Job drawing, mm, ordinate dimensions from the low corner. One solid piece. A direction names the side the tool comes from. Give positions to 0.01 mm unless a question says otherwise; leave off trailing zeros. Loops run counter-clockwise (first coordinate to the right, second up) from the corner with the lowest first, then second, coordinate; pieces in that order, holes last. Notation, with made-up numbers: M 77,42.25 L 88,42.25 A30 ccw 88,68.25 Z; hole C -30,1.25 d9. An arc over 180 degrees is marked long. One line per question, with ' | ' between items.
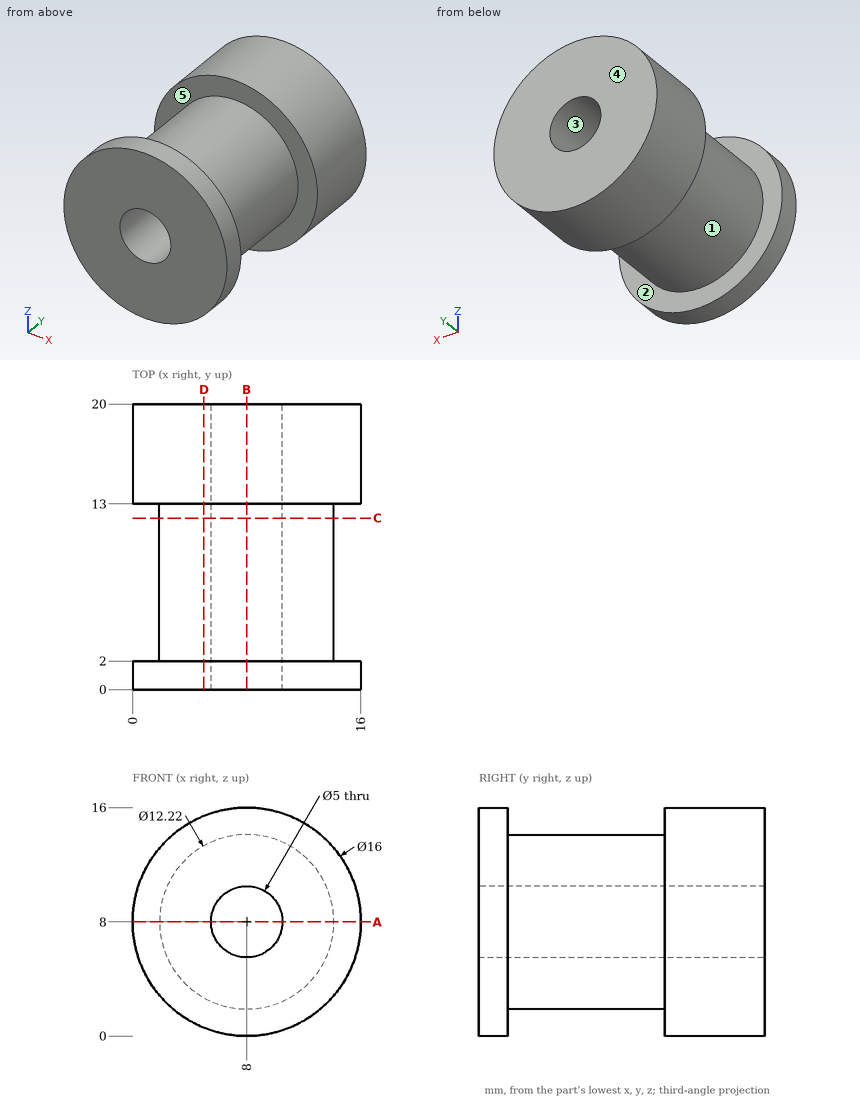
Item 1: Saw through at C-C on y = 12. Give the cut face in (x, z).
Conclusion:
outline: C 8,8 d12.22; hole C 8,8 d5
Item 2: Saw through at A-A on z = 8. Give the cut face in (x, y).
Conclusion:
outline: M 0,0 L 5.5,0 L 5.5,20 L 0,20 L 0,13 L 1.89,13 L 1.89,2 L 0,2 Z; M 10.5,0 L 16,0 L 16,2 L 14.11,2 L 14.11,13 L 16,13 L 16,20 L 10.5,20 Z
Item 3: Saw through at D-D on x = 5. Give the cut face in (y, z).
Conclusion:
outline: M 0,0.58 L 2,0.58 L 2,2.68 L 13,2.68 L 13,0.58 L 20,0.58 L 20,15.42 L 13,15.42 L 13,13.32 L 2,13.32 L 2,15.42 L 0,15.42 Z
Item 4: 3-axis set-ups, long thin cutter, end or side, ignore diameter. For the marked faces 4 and 5: which of +Z, -Z, +X, -X, +Y, -Y reach the whole face in a straight line?
Conclusion:
face 4: +Z, -Z, +X, -X, +Y | face 5: none
Item 5: Mould opens along X. For the marked faces 1, 2 and 3 say: pulls with the +X half, pulls with the -X half, needs draft (parallel to the pull), parting line crosses it, or undercut.
Conclusion:
face 1: parting line crosses it | face 2: needs draft | face 3: undercut
Item 6: Saw through at B-B on x = 8. Give the cut face in (y, z).
Conclusion:
outline: M 0,0 L 2,0 L 2,1.89 L 13,1.89 L 13,0 L 20,0 L 20,5.5 L 0,5.5 Z; M 0,10.5 L 20,10.5 L 20,16 L 13,16 L 13,14.11 L 2,14.11 L 2,16 L 0,16 Z
Item 7: Drill centre lines: line 1 along Y through (x, z) = (10, 0.5); line 2 along X through (y, z) = (15.5, 8); line 3 along X through (y, z) = (6, 8). Where is each one in solid material? Low to high. Write a range as [from, to].
Conclusion:
line 1: [0, 2], [13, 20] | line 2: [0, 5.5], [10.5, 16] | line 3: [1.89, 5.5], [10.5, 14.11]
Item 8: Drop flat-ended pins along their axis: P1, Ø4, axis at x = 5.5, y = 9.5, coming from the +Z side; P2, Ø4.5, axis at x = 8, z = 8, coming from the -Y side; P3, Ø6, axis at y = 7.5, z = 13.5, coming from the -X side; P4, Ø5, axis at x = 4.5, y = 10, coming from the -Z side. Give the stop position or say it passes through.
Conclusion:
P1: z = 14.09 | P2: through | P3: x = 2.42 | P4: z = 1.97
